Source: CAD feature listing. Evaluate the final solid. Frame: model axes, mm. Face numbers are marked on the shaded views. A direction names the side the tool comes from. Give positions to 0.01 mm unless a question says otherwise; leave off trailing zeros.
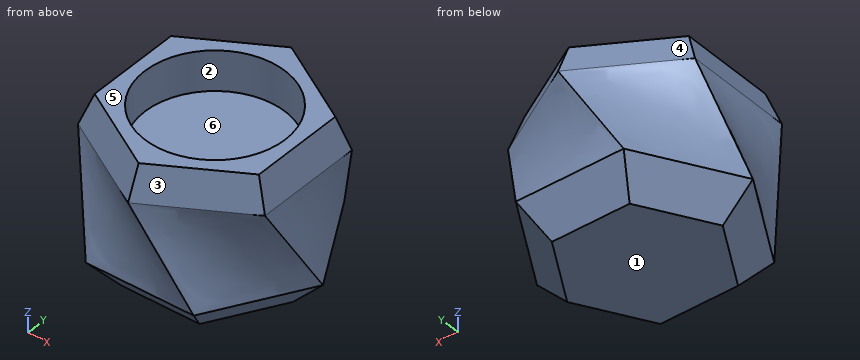
from build123d import *

# Parameters (mm, degrees)
F4_DEPTH = 10
F4_TAPER = 40
F5_DEPTH = 10
F5_TAPER = 20
F6_R     = 22.5
F7_DEPTH = 12.8


with BuildPart() as f3:
    # F0 (on Top) → F3 section 0
    with BuildSketch(Plane.XY):
        Polygon((34.6410161514, 0), (17.3205080757, 30), (-17.3205080757, 30), (-34.6410161514, 0), (-17.3205080757, -30), (17.3205080757, -30), align=None)
    # F2 (on offset) → F3 section 1
    with BuildSketch(Plane.XY.offset(30)):
        Polygon((0, 34.6410161514), (-30, 17.3205080757), (-30, -17.3205080757), (0, -34.6410161514), (30, -17.3205080757), (30, 17.3205080757), align=None)
    loft()

    # F3_face (on face) → F4 (join)
    with BuildSketch(Plane(origin=(0, 0, 0), x_dir=(1, 0, 0), z_dir=(0, 0, -1))):
        Polygon((17.3205080757, 30), (-17.3205080757, 30), (-34.6410161514, 0), (-17.3205080757, -30), (17.3205080757, -30), (34.6410161514, 0), align=None)
    extrude(amount=F4_DEPTH, taper=F4_TAPER)

    # F3_face1 (on face) → F5 (join)
    with BuildSketch(Plane.XY.offset(30)):
        Polygon((0, -34.6410161514), (30, -17.3205080757), (30, 17.3205080757), (0, 34.6410161514), (-30, 17.3205080757), (-30, -17.3205080757), align=None)
    extrude(amount=F5_DEPTH, taper=F5_TAPER)

    # F6 (on face) → F7 (cut)
    with BuildSketch(Plane.XY.offset(40)):
        Circle(F6_R)
    extrude(amount=-F7_DEPTH, mode=Mode.SUBTRACT)


solid = f3.part
1) Ray query, probe 1 along Y at (x, z) = (0, 30); probe 2 along Z at (x, y) = (-17, 0); probe 3 along Y at (x, z) = (0, 36.5). Return the intervals inside material, ascending.
Checks:
probe 1: y = -34.64 to -22.5, 22.5 to 34.64
probe 2: z = -10 to 27.2
probe 3: y = -31.91 to -22.5, 22.5 to 31.91
2) Pull-direction query (Y, two-part tool) for the marked faces 1, 2, 3 and 4; classes: released by +Y, released by -Y, zero draft, split by the parting line, or undercut.
Checks:
face 1: zero draft
face 2: undercut
face 3: released by -Y
face 4: released by +Y
3) Reachability of the marked faces 5 and 6 from +Z, -Z, +X, -X, +Y, -Y: full face, straight path, thin tool, end or side. Return the list, or none.
Checks:
face 5: +Z, +X, -X, +Y, -Y
face 6: +Z
4) Contact query for flat-ended pins moving along their axis: P1, Ø13.5, axis at x = -6.5, y = 10.5, coming from the +Z side; P2, Ø8, axis at x = 21, z = 14, coming from the +Y side; P3, Ø1.5, axis at x = -1.5, z = 13, coming from the +Y side. Output: stop coordinate, or through.
Checks:
P1: stops at z = 27.2
P2: stops at y = 26.06
P3: stops at y = 30.3
